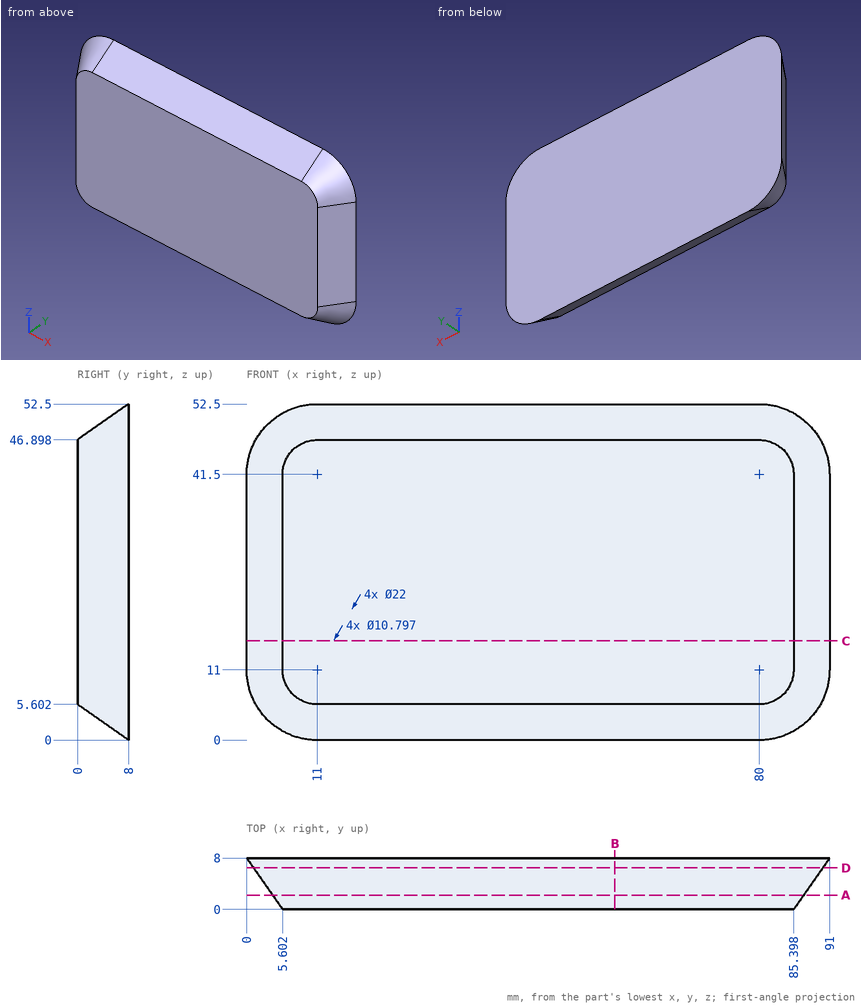
Could you check a few things on this drawing? It's one solid part, dimensions in mm from its lowest x, y, z. Round coordinates to 2 decimals unless told otherwise and drop trailing zeros. Write each loop counter-clockwise with the first axis right and the second up, starting at its lowest first coordinate (ties: lowest second). Pieces come first, ordered by that corner, then holes. Notation, with made-up numbers: (24.5, -6.5) -> (78.5, -6.5) arc R25 ccw to (78.5, 30.5) -> close; hole circle Ø1 at (-38.75, -38.5). An arc over 180 degrees is marked (long way). Use a Markdown table: item, result.
1. Please list where these lines run through material, in increasing order: probe 1 along X at (y, z) = (2.75, 38.5) (1 decimal); probe 2 along Z at (x, y) = (71, 5.25) (1 decimal); probe 3 along Z at (x, y) = (63, 3.5).
Answer key:
| item | result |
|---|---|
| probe 1 | x = 3.7 to 87.3 |
| probe 2 | z = 1.9 to 50.6 |
| probe 3 | z = 3.15 to 49.35 |
2. If we section it at C-C (z = 15.5): List the corners of the cut face in (x, y) for me.
Answer key:
| item | result |
|---|---|
| outline | (0, 8) -> (5.6, 0) -> (85.4, 0) -> (91, 8) -> close |
3. If we section it at A-A (y = 2.25): List the corners of the cut face in (x, z) for me.
Answer key:
| item | result |
|---|---|
| outline | (4.03, 11) arc R6.97 ccw to (11, 4.03) -> (80, 4.03) arc R6.97 ccw to (86.97, 11) -> (86.97, 41.5) arc R6.97 ccw to (80, 48.47) -> (11, 48.47) arc R6.97 ccw to (4.03, 41.5) -> close |
4. If we section it at B-B (x = 57.5): List the corners of the cut face in (y, z) for me, then the cut area to 3 significant figures.
Answer key:
| item | result |
|---|---|
| outline | (0, 5.6) -> (8, 0) -> (8, 52.5) -> (0, 46.9) -> close |
| area | 375 mm^2 |
5. If we section it at D-D (y = 6.5): List the corners of the cut face in (x, z) for me, then the cut area to 3 significant figures.
Answer key:
| item | result |
|---|---|
| outline | (1.05, 11) arc R9.95 ccw to (11, 1.05) -> (80, 1.05) arc R9.95 ccw to (89.95, 11) -> (89.95, 41.5) arc R9.95 ccw to (80, 51.45) -> (11, 51.45) arc R9.95 ccw to (1.05, 41.5) -> close |
| area | 4,400 mm^2 |
6. For pin 1 Ø3 at (y, z) = (7, 6) entering from +X; pin 2 Ø1 at (y, z) = (1.5, 6.5) entering from -X; pin 3 Ø3 at (y, z) = (1.5, 36.5) entering from +X, each with a flat end and sliding along its axis, tell me the tip position at first contact or that it passes through.
Answer key:
| item | result |
|---|---|
| pin 1 | stops at x = 90.29 |
| pin 2 | stops at x = 5.74 |
| pin 3 | stops at x = 87.5 |
